Work out the finished part from the listing and answer in its coordinate system (mm). Round coordinates to 2 decimals unless told otherwise and drop trailing zeros. Order: outer loops, then holes, each group sorted by start corner. A loop starts at its lowest first (then second) coordinate and runs counter-clockwise, first axis right, second up. Notation, with made-up numbers: (28, -36.5) -> (54, -36.5) arc R29 cw to (54, -4.5) -> close; hole circle Ø7 at (-31.5, 67.5). An arc over 180 degrees is marked (long way). Use a Markdown table: item, result. Add a question column.
Item 1: Find the intervals of material crossed by L1, parallel to X at y = 1.5, z = -38.1; L2, parallel to Z at x = 8, y = 5.5; L3, parallel to Z at x = 7.5, y = 4.75, in increasing order. Write a range as [from, to].
Item 2: A cutting plane is placed at B-B, the plane y = 1.5. Determine the outline of the cut face in (x, z), plus the area to 3 significant figures.
Item 3: A flat-ended cylindrical pin translates along its axis: P1, Ø6.5, axis at x = 9.398, z = -12.7, coming from the +Y side. Find the tip coordinate at first contact, or state that the pin passes through.
Item 4: A cutting plane is placed at A-A, the plane z = -12.7. Determine the outline of the cut face in (x, y), plus the area to 3 significant figures.
Item 5: A cutting plane is placed at D-D, the plane y = 5. Determine the outline of the cut face in (x, z).
Item 6: A cutting plane is placed at C-C, the plane x = 9.5. Give the number of separate pieces and of enclosed holes in the cut face, plus the area to 3 significant figures.
Item 7: For a pull along X with two mould halves and no side action, classify faces 1 (the flat face through (18.796, 3, -25)), 2 (the flat face through (0, 3, -25)), 3 (the flat face through (9, 6.35, -26)), 4 (the conical face through (8.2, 4.5, -10.3)) as +X half, -X half, draft (parallel to the pull), parting line (faces both ways), or undercut.
from build123d import *

# Parameters (mm, degrees)
SKETCH1_W                                          = 18.796
SKETCH1_H                                          = 50.8
BOSS_EXTRUDE1_DEPTH                                = 6.35
CSK_FOR_10_FLAT_HEAD_MACHINE_SCREW_100_D           = 5.1054
CSK_FOR_10_FLAT_HEAD_MACHINE_SCREW_100_DEPTH       = 25.4
CSK_FOR_10_FLAT_HEAD_MACHINE_SCREW_100_CSINK_D     = 9.779
CSK_FOR_10_FLAT_HEAD_MACHINE_SCREW_100_CSINK_ANGLE = 100
CSK_FOR_10_FLAT_HEAD_MACHINE_SCREW_100_TIP         = 1.533816902


with BuildPart() as part:
    # Sketch1 → Boss-Extrude1 (new body)
    with BuildSketch(Plane(origin=(0, 0, 0), x_dir=(1, 0, 0), z_dir=(0, 1, 0))):
        with Locations((9.398, 25.4)):
            Rectangle(SKETCH1_W, SKETCH1_H)
    extrude(amount=BOSS_EXTRUDE1_DEPTH)

    # CSK for #10 Flat Head Machine Screw (100)1
    with Locations(Plane(origin=(0, 6.35, 0), x_dir=(1, 0, 0), z_dir=(0, 1, 0))):
        with Locations((9.398, 38.1), (9.398, 12.7)):
            CounterSinkHole(CSK_FOR_10_FLAT_HEAD_MACHINE_SCREW_100_D / 2, CSK_FOR_10_FLAT_HEAD_MACHINE_SCREW_100_CSINK_D / 2, depth=CSK_FOR_10_FLAT_HEAD_MACHINE_SCREW_100_DEPTH, counter_sink_angle=CSK_FOR_10_FLAT_HEAD_MACHINE_SCREW_100_CSINK_ANGLE)
            with Locations((0, 0, -(CSK_FOR_10_FLAT_HEAD_MACHINE_SCREW_100_DEPTH + CSK_FOR_10_FLAT_HEAD_MACHINE_SCREW_100_TIP / 2))):  # 118° drill point
                Cone(0, CSK_FOR_10_FLAT_HEAD_MACHINE_SCREW_100_D / 2, CSK_FOR_10_FLAT_HEAD_MACHINE_SCREW_100_TIP, mode=Mode.SUBTRACT)


solid = part.part
Reported:
| question | item | result |
|---|---|---|
| 1 | L1 | [0, 6.85], [11.95, 18.8] |
| 1 | L2 | [-50.8, -41.72], [-34.48, -16.32], [-9.08, 0] |
| 1 | L3 | [-50.8, -40.4], [-35.8, -15], [-10.4, 0] |
| 2 | outline | (0, -50.8) -> (18.8, -50.8) -> (18.8, 0) -> (0, 0) -> close; hole circle Ø5.11 at (9.4, -38.1); hole circle Ø5.11 at (9.4, -12.7) |
| 2 | area | 914 mm² |
| 3 | P1 | y = 4.97 |
| 4 | outline | (0, 0) -> (6.85, 0) -> (6.85, 4.39) -> (4.51, 6.35) -> (0, 6.35) -> close; (11.95, 0) -> (18.8, 0) -> (18.8, 6.35) -> (14.29, 6.35) -> (11.95, 4.39) -> close |
| 4 | area | 82.4 mm² |
| 5 | outline | (0, -50.8) -> (18.8, -50.8) -> (18.8, 0) -> (0, 0) -> close; hole circle Ø6.56 at (9.4, -38.1); hole circle Ø6.56 at (9.4, -12.7) |
| 6 | separate pieces | 3 |
| 6 | enclosed holes | 0 |
| 6 | area | 249 mm² |
| 7 | face 1 | +X half |
| 7 | face 2 | -X half |
| 7 | face 3 | draft |
| 7 | face 4 | undercut |
